Can you work these out from the model? Positions are in its coordinate system, mm. Face numbers are marked on the shaded views. A direction names the side the tool comes from. Give positions to 0.01 mm unless a question says otherwise; leave off trailing zeros. Order: outer loops, then holes, each group sorted by start corner. A loop starts at its lowest first (then second) coordinate and runs counter-clockwise, first axis right, second up. Notation, with made-up numbers: (47, 46.5) -> (88, 46.5) arc R32 cw to (88, 80.5) -> close; hole circle Ø11 at (80, 28). An arc over 180 degrees is marked (long way). Answer as a JSON object with one key per item and string values.
```python
from build123d import *

# Parameters (mm, degrees)
SKETCH1_R            = 40
SKETCH1_R_2          = 12.5
BOSS_EXTRUDE1_DEPTH  = 6
SKETCH2_R            = 20
SKETCH2_R_2          = 12.5
BOSS_EXTRUDE2_DEPTH  = 30
SKETCH6_R            = 20
SKETCH6_R_2          = 16.25
BOSS_EXTRUDE5_DEPTH  = 12
BOSS_EXTRUDE6_DEPTH  = 42
SKETCH9_R            = 17.6
CUT_EXTRUDE1_DEPTH   = 3
BOSS_EXTRUDE14_START = -6
SKETCH11_R           = 40
SKETCH11_R_2         = 20
BOSS_EXTRUDE14_DEPTH = 6
SKETCH12_R           = 3
CUT_EXTRUDE2_DEPTH   = 78


with BuildPart() as part:
    # Sketch1 → Boss-Extrude1 (new body)
    with BuildSketch(Plane.XY):
        Circle(SKETCH1_R)
        Circle(SKETCH1_R_2, mode=Mode.SUBTRACT)
    extrude(amount=BOSS_EXTRUDE1_DEPTH)

    # Sketch2 → Boss-Extrude2 (add)
    with BuildSketch(Plane.XY.offset(6)):
        Circle(SKETCH2_R)
        Circle(SKETCH2_R_2, mode=Mode.SUBTRACT)
    extrude(amount=BOSS_EXTRUDE2_DEPTH)

    # Sketch6 → Boss-Extrude5 (add)
    with BuildSketch(Plane.XY.offset(36)):
        Circle(SKETCH6_R)
        Circle(SKETCH6_R_2, mode=Mode.SUBTRACT)
    extrude(amount=BOSS_EXTRUDE5_DEPTH)

    # Sketch8 → Boss-Extrude6 (add)
    with BuildSketch(Plane.XY.offset(6)):
        with BuildLine():
            Line((4, -39.799497484), (4, -19.595917942))
            ThreePointArc((4, -19.595917942), (0, -20), (-4, -19.595917942))
            Line((-4, -19.595917942), (-4, -39.799497484))
            ThreePointArc((-4, -39.799497484), (0, -40), (4, -39.799497484))
        make_face()
        with BuildLine():
            Line((39.799497484, 4), (19.595917942, 4))
            ThreePointArc((19.595917942, 4), (20, 0), (19.595917942, -4))
            Line((19.595917942, -4), (39.799497484, -4))
            ThreePointArc((39.799497484, -4), (40, 0), (39.799497484, 4))
        make_face()
        with BuildLine():
            Line((-39.799497484, -4), (-19.595917942, -4))
            ThreePointArc((-19.595917942, -4), (-20, 0), (-19.595917942, 4))
            Line((-19.595917942, 4), (-39.799497484, 4))
            ThreePointArc((-39.799497484, 4), (-40, 0), (-39.799497484, -4))
        make_face()
        with BuildLine():
            Line((-4, 39.799497484), (-4, 19.595917942))
            ThreePointArc((-4, 19.595917942), (0, 20), (4, 19.595917942))
            Line((4, 19.595917942), (4, 39.799497484))
            ThreePointArc((4, 39.799497484), (0, 40), (-4, 39.799497484))
        make_face()
    extrude(amount=BOSS_EXTRUDE6_DEPTH)

    # Sketch9 → Cut-Extrude1 (cut)
    with BuildSketch(Plane.XY.offset(48)):
        Circle(SKETCH9_R)
    extrude(amount=-CUT_EXTRUDE1_DEPTH, mode=Mode.SUBTRACT)

    # Sketch11 → Boss-Extrude14 (add)
    with BuildSketch(Plane.XY.offset(48).offset(BOSS_EXTRUDE14_START)):
        Circle(SKETCH11_R)
        Circle(SKETCH11_R_2, mode=Mode.SUBTRACT)
    extrude(amount=BOSS_EXTRUDE14_DEPTH)

    # Sketch12 → Cut-Extrude2 (cut)
    with BuildSketch(Plane(origin=(0, 0, 0), x_dir=(-1, 0, 0), z_dir=(0, 0, -1))):
        with Locations(Location((-21.213203436, 21.213203436, 0), (0, 0, 180))):
            Circle(SKETCH12_R)
        with Locations(Location((21.213203436, 21.213203436, 0), (0, 0, 180))):
            Circle(SKETCH12_R)
        with Locations(Location((21.213203436, -21.213203436, 0), (0, 0, 180))):
            Circle(SKETCH12_R)
        with Locations(Location((-21.213203436, -21.213203436, 0), (0, 0, 180))):
            Circle(SKETCH12_R)
    extrude(amount=-CUT_EXTRUDE2_DEPTH, mode=Mode.SUBTRACT)


solid = part.part
```
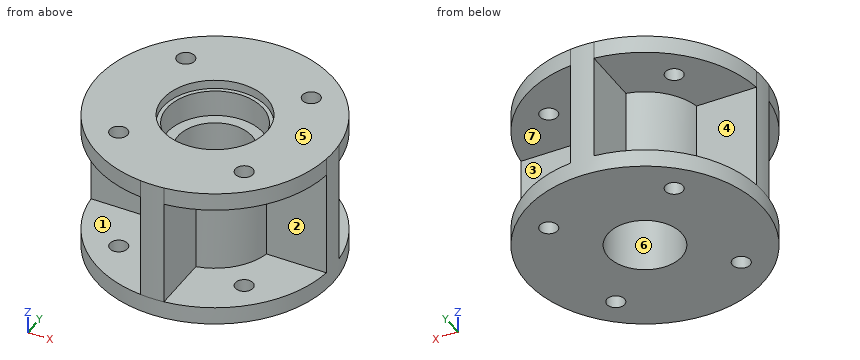
1. If we mould it in two halves opening along Z, with no side actions, what happens to the marked faces 5, 6 and 7? For each: +Z half, -Z half, draft (parallel to the pull), parting line (faces both ways), or undercut.
Worked answers:
{"face 5": "+Z half", "face 6": "draft", "face 7": "undercut"}
2. Please list where these lines run through material, in increasing order: L1, parallel to Z at x = 33, y = 5.5; L2, parallel to Y at x = -26, z = 32.
Worked answers:
{"L1": "0 to 6, 42 to 48", "L2": "-4 to 4"}
3. Will these pins go through, and if not, where does the flat tip stop? pin 1 Ø3 at (x, z) = (-1.5, 32) entering from +Y; pin 2 Ø3 at (x, z) = (-28.5, 31) entering from +Y; pin 3 Ø6 at (y, z) = (31, 21) entering from -X; pin 4 Ø1 at (x, y) = (9.5, -5) entering from -Z.
Worked answers:
{"pin 1": "y = 40", "pin 2": "y = 4", "pin 3": "x = -4", "pin 4": "through"}
4. If we section it at D-D on x = 28: Please give me the cut outline in (y, z).
Worked answers:
{"outline": "(-28.57, 0) -> (28.57, 0) -> (28.57, 6) -> (4, 6) -> (4, 42) -> (28.57, 42) -> (28.57, 48) -> (-28.57, 48) -> (-28.57, 42) -> (-4, 42) -> (-4, 6) -> (-28.57, 6) -> close"}
5. If we section it at A-A on y = 0: Please give me the cut outline in (x, z), then the cut area to 3 significant figures.
Worked answers:
{"outline": "(-40, 0) -> (-12.5, 0) -> (-12.5, 36) -> (-16.25, 36) -> (-16.25, 45) -> (-17.6, 45) -> (-17.6, 48) -> (-40, 48) -> close; (12.5, 0) -> (40, 0) -> (40, 48) -> (17.6, 48) -> (17.6, 45) -> (16.25, 45) -> (16.25, 36) -> (12.5, 36) -> close", "area": "2,540 mm²"}
6. For the marked faces 1, 2, 3 and 4, which set-ups out of +Z, -Z, +X, -X, +Y, -Y let a thin tool reach every point of the face, with its end or its side?
Worked answers:
{"face 1": "-X, -Y", "face 2": "+X, -Y", "face 3": "+X, +Y", "face 4": "-X, +Y"}
7. If we section it at C-C on z = 38: Please give me the cut outline in (x, y).
Worked answers:
{"outline": "(-39.8, -4) -> (-19.6, -4) arc R20 ccw to (-4, -19.6) -> (-4, -39.8) arc R40 ccw to (4, -39.8) -> (4, -19.6) arc R20 ccw to (19.6, -4) -> (39.8, -4) arc R40 ccw to (39.8, 4) -> (19.6, 4) arc R20 ccw to (4, 19.6) -> (4, 39.8) arc R40 ccw to (-4, 39.8) -> (-4, 19.6) arc R20 ccw to (-19.6, 4) -> (-39.8, 4) arc R40 ccw to start; hole circle Ø32.5 at (0, 0)"}
